Study the drawing (mm; zero at the part's minimum x, y, z) and answer. A direction names the side the tool comes from. Coordinates: 2 decimals unless noted, no trailing zeros. Loops run counter-clockwise (first coordinate to the right, second up) from the corner with the lowest first, then second, coordinate; pieces in that order, holes last. Notation, with made-up numbers: (-40, 1) -> (-34, 1) arc R19 ccw to (-34, 20) -> close; hole circle Ø9 at (88.25, 17.25). An arc over 180 degrees is marked (long way). Answer in a Markdown table with one row per item.
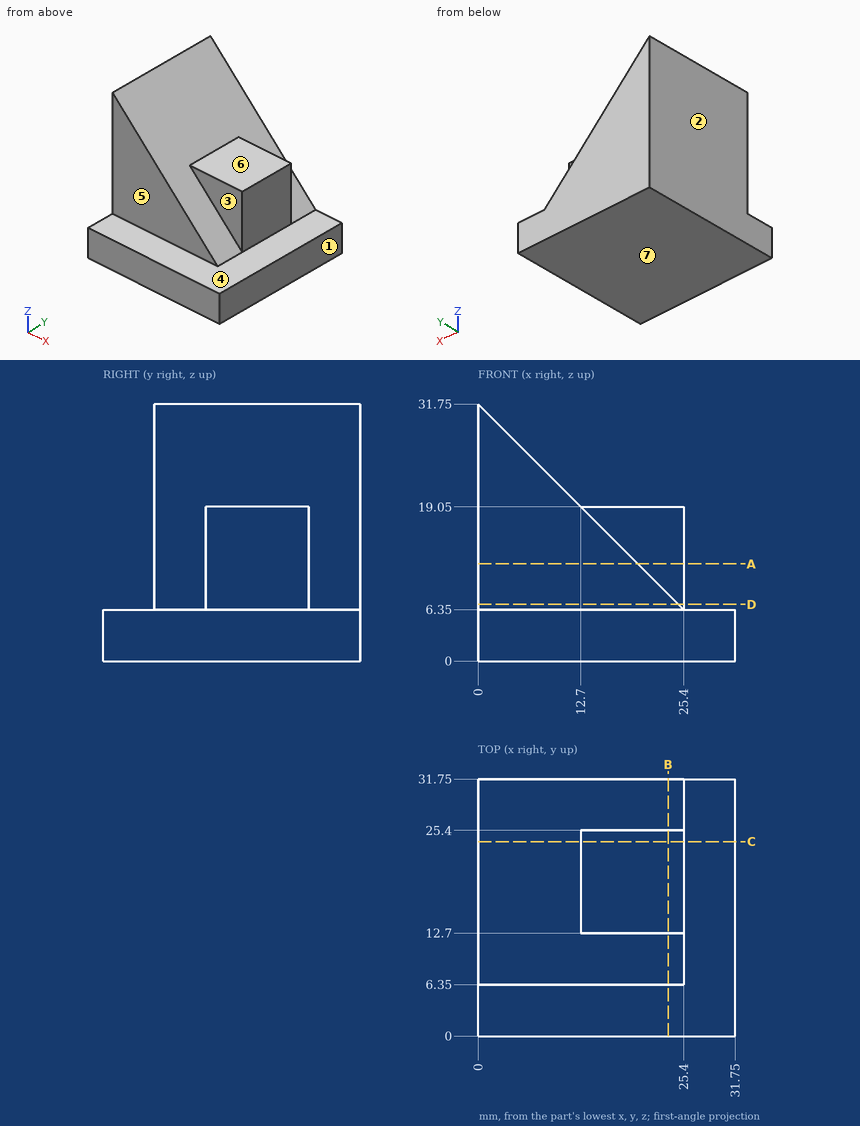
1. The mould has two halves that part along X. Classify the marked faces 1, 2 and 3: pulls with the +X half, pulls with the -X half, needs draft (parallel to the pull), parting line crosses it, or undercut.
A:
| item | result |
|---|---|
| face 1 | pulls with the +X half |
| face 2 | pulls with the -X half |
| face 3 | needs draft |
2. A tool of negligible diameter and unlimited length cuts with its end or side. For the marked faces 4, 5, 6 and 7, from which of +Z, -Z, +X, -X, +Y, -Y can it reach the whole face along a straight path? Write none if from no direction.
A:
| item | result |
|---|---|
| face 4 | +Z, +X, -Y |
| face 5 | +Z, +X, -X, -Y |
| face 6 | +Z, +X, +Y, -Y |
| face 7 | -Z, +X, -X, +Y, -Y |
3. Find the intervals of material crossed by probe 1 along Y at (x, z) = (12.5, 19); probe 2 along X at (y, z) = (23, 13.5); probe 3 along Z at (x, y) = (29, 23.5), in increasing order.
A:
| item | result |
|---|---|
| probe 1 | y = 6.35 to 31.75 |
| probe 2 | x = 0 to 25.4 |
| probe 3 | z = 0 to 6.35 |
4. A cutting plane is placed at B-B on x = 23.5. Give the vertices of the cut face in (y, z), and give its area (3 significant figures).
A:
| item | result |
|---|---|
| outline | (0, 0) -> (31.75, 0) -> (31.75, 8.25) -> (25.4, 8.25) -> (25.4, 19.05) -> (12.7, 19.05) -> (12.7, 8.25) -> (6.35, 8.25) -> (6.35, 6.35) -> (0, 6.35) -> close |
| area | 387 mm2 |
5. Given pin 1 Ø6.5 at (x, z) = (21, 14.5) entering from +Y; pin 2 Ø2 at (y, z) = (7, 22) entering from +X; pin 3 Ø4 at (x, y) = (16, 21.5) entering from +Z; pin 4 Ø10 at (x, z) = (26.5, 23.5) entering from +Y, each flat-ended and moving along its own axis, determine where each tip first touches the part or whether it passes through.
A:
| item | result |
|---|---|
| pin 1 | stops at y = 31.75 |
| pin 2 | stops at x = 10.75 |
| pin 3 | stops at z = 19.05 |
| pin 4 | stops at y = 25.4 |
6. A cutting plane is placed at C-C on y = 24. Give the vertices of the cut face in (x, z), and give its area (3 significant figures).
A:
| item | result |
|---|---|
| outline | (0, 0) -> (31.75, 0) -> (31.75, 6.35) -> (25.4, 6.35) -> (25.4, 19.05) -> (12.7, 19.05) -> (0, 31.75) -> close |
| area | 605 mm2 |
7. A cutting plane is placed at D-D on z = 7. Give the vertices of the cut face in (x, y).
A:
| item | result |
|---|---|
| outline | (0, 6.35) -> (24.75, 6.35) -> (24.75, 12.7) -> (25.4, 12.7) -> (25.4, 25.4) -> (24.75, 25.4) -> (24.75, 31.75) -> (0, 31.75) -> close |
8. A cutting plane is placed at A-A on z = 12. Give the vertices of the cut face in (x, y).
A:
| item | result |
|---|---|
| outline | (0, 6.35) -> (19.75, 6.35) -> (19.75, 12.7) -> (25.4, 12.7) -> (25.4, 25.4) -> (19.75, 25.4) -> (19.75, 31.75) -> (0, 31.75) -> close |
